from build123d import *

# Parameters (mm, degrees)
SKETCH2_R          = 1.25
CUT_EXTRUDE1_DEPTH = 15.302796929


with BuildPart() as part:
    # Sketch1 → Revolve1 (revolve)
    with BuildSketch(Plane.XY, mode=Mode.PRIVATE) as revolve1_sk:
        Polygon((1.6, 3), (1.6, 4.5), (9.35, 4.5), (9.6, 4.25), (9.6, 2.25), (9.35, 2), (5.3, 2), (5.3, 0.25), (5.05, 0), (2.6, 0), (2.6, 3), align=None)
    revolve(revolve1_sk.sketch.rotate(Axis((0, 0, 0), (0, 1, 0)), 90), axis=Axis((0, 0, 0), (0, 1, 0)))

    # Sketch2 → Cut-Extrude1 (cut, through all)
    with BuildSketch(Plane(origin=(0, 0, 0), x_dir=(1, 0, 0), z_dir=(0, 1, 0))):
        with Locations(Location((0, 7, 0), (0, 0, 90))):
            Circle(SKETCH2_R)
        with Locations(Location((0, -7, 0), (0, 0, 90))):
            Circle(SKETCH2_R)
        with Locations(Location((7, 0, 0), (0, 0, 90))):
            Circle(SKETCH2_R)
        with Locations(Location((-7, 0, 0), (0, 0, 90))):
            Circle(SKETCH2_R)
    extrude(amount=CUT_EXTRUDE1_DEPTH, mode=Mode.SUBTRACT)


solid = part.part
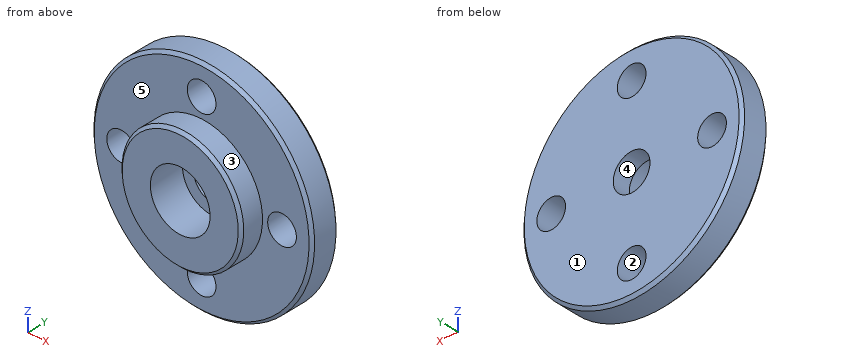
Input: part model. Units: mm. Frame: model coordinates. Face numbers are marked on the shaded views. A direction names the side the tool comes from. Give positions to 0.01 mm unless a question says otherwise; leave off trailing zeros. Write each loop counter-clockwise with the first axis right and the second up, starting at its lowest first coordinate (ties: lowest second). Pieces come first, ordered by that corner, then holes. Notation, with made-up numbers: (81, 73) -> (119, 73) arc R14 ccw to (119, 98) -> close; hole circle Ø7 at (82, -24.5). An arc over 180 degrees is marked (long way). Use one line per item in the form item = value. Start each with the question number.
1) Pin query (flat end, axial travel): pin 1 (2 mm diameter, centred on x = -1.5, y = 2, fed in from +Z); pin 2 (1.5 mm diameter, centred on x = -7, z = 0, fed in from +Y); pin 3 (1.5 mm diameter, centred on y = 1, z = -5.5, fed in from +X); pin 4 (2 mm diameter, centred on y = 3, z = 3, fed in from -X). Return the tip coordinate at first contact, or that it passes through.
2) Draft query along X for the marked faces 1, 2 and 3. Return one class per face: pulls with the +X half, pulls with the -X half, needs draft (parallel to the pull), parting line crosses it, or undercut.
3) Ray query, probe 1 along X at (y, z) = (3.2, 0); probe 2 along X at (y, z) = (1, 0); probe 3 along Y at (x, z) = (5, 3). Return the intervals inside material, ascending. Write a range as from..to.
4) Section query A-A on x = 0. Count the separate pieces of the cut face and the enclosed holes in it, then the cut area to 3 significant figures.
5) Section query B-B on y = 2.7. Return the cut outline in (x, z).
6) Set-up query: the marked faces 4 and 5. Return all of +Z, -Z, +X, -X, +Y, -Y with unobstructed straight access to the full face (end or side cutting, diameter ignored); none if empty.
7) Section query D-D on y = 1.7. Return the cut outline in (x, z), then the cut area to 3 significant figures.
Outcome:
q1.pin_1 = 9.59
q1.pin_2 = through
q1.pin_3 = 2.35
q1.pin_4 = -9.39
q2.face_1 = needs draft
q2.face_2 = undercut
q2.face_3 = parting line crosses it
q3.probe_1 = -9.6..-8.25, -5.75..-1.6, 1.6..5.75, 8.25..9.6
q3.probe_2 = -5.3..-2.6, 2.6..5.3
q3.probe_3 = 2..4.5
q4.separate_pieces = 4
q4.enclosed_holes = 0
q4.area = 36.1 mm^2
q5.outline = circle Ø19.2 at (0, 0); hole circle Ø2.5 at (-7, 0); hole circle Ø5.2 at (0, 0); hole circle Ø2.5 at (0, -7); hole circle Ø2.5 at (0, 7); hole circle Ø2.5 at (7, 0)
q6.face_4 = +Y, -Y
q6.face_5 = -Y
q7.outline = circle Ø10.6 at (0, 0); hole circle Ø5.2 at (0, 0)
q7.area = 67.0 mm^2
